Work out the finished part from the listing and answer in its coordinate system (mm). A direction names the side the tool comes from. Round coordinates to 2 decimals unless told otherwise and drop trailing zeros. Loops run counter-clockwise (first coordinate to the right, second up) from the corner with the lowest first, then second, coordinate; pieces in that order, holes last. Notation, with made-up numbers: (69, 23) - (75, 23) arc R16 cw to (75, 34) - close; hole circle Ø5 at (32.25, 22.25). An arc over 180 degrees is marked (long way). Return JSON: item names as keys, results as strings.
from build123d import *

# Parameters (mm, degrees)
F0_W     = 10
F0_H     = 20
F1_DEPTH = 1.5
F2_W     = 10
F2_H     = 1.5
F3_DEPTH = 18.5
F5_DEPTH = 1.501
F7_DEPTH = 1.501
F9_DEPTH = 1
F10_R    = 0.99999


# Not quite as in the source:
# - a fillet or chamfer is up to 0.001 mm smaller than in the source, because OpenCascade refuses the exact size
# - a pattern or mirror of a feature is missing from the dataset's text; its kind, count and spacing are read off the source's solid


with BuildPart() as f1:
    # F0 (on Top) → F1 (new body)
    with BuildSketch(Plane.XY):
        Rectangle(F0_W, F0_H)
    extrude(amount=F1_DEPTH)

    # F2 (on face) → F3 (join)
    with BuildSketch(Plane.XY.offset(1.5)):
        with Locations((0, 9.25)):
            Rectangle(F2_W, F2_H)
    extrude(amount=F3_DEPTH)

    # F4 (on face) → F5 (cut, through all)
    with BuildSketch(Plane.XY.offset(1.5)):
        with BuildLine():
            ThreePointArc((0, -5), (1.2727922061, -4.4727922061), (1.8, -3.2))
            Line((1.8, -3.2), (1.8, 3.2))
            ThreePointArc((1.8, 3.2), (1.2727922061, 4.4727922061), (0, 5))
            ThreePointArc((0, 5), (-1.2727922061, 4.4727922061), (-1.8, 3.2))
            Line((-1.8, 3.2), (-1.8, -3.2))
            ThreePointArc((-1.8, -3.2), (-1.2727922061, -4.4727922061), (0, -5))
        make_face()
    extrude(amount=-F5_DEPTH, mode=Mode.SUBTRACT)

    # F6 (on face) → F7 (cut, through all)
    with BuildSketch(Plane.XZ.offset(-8.5)):
        with BuildLine():
            ThreePointArc((0, 4.6788305809), (1.2727922061, 5.2060383747), (1.8, 6.4788305809))
            Line((1.8, 6.4788305809), (1.8, 12.8788305809))
            ThreePointArc((1.8, 12.8788305809), (1.2727922061, 14.151622787), (0, 14.6788305809))
            ThreePointArc((0, 14.6788305809), (-1.2727922061, 14.151622787), (-1.8, 12.8788305809))
            Line((-1.8, 12.8788305809), (-1.8, 6.4788305809))
            ThreePointArc((-1.8, 6.4788305809), (-1.2727922061, 5.2060383747), (0, 4.6788305809))
        make_face()
    extrude(amount=-F7_DEPTH, mode=Mode.SUBTRACT)

    # F8 (on face) → F9 (join)
    with BuildSketch(Plane(origin=(-5, 0, 0), x_dir=(0, -1, 0), z_dir=(-1, 0, 0))):
        Polygon((10, 1.5), (-8.5, 20), (-8.5, 1.5), align=None)
    f9 = extrude(amount=-F9_DEPTH)

    # F9_copies: F9 across plane
    add(f9.mirror(Plane(origin=(0, 0, 0), x_dir=(0, 0, 1), z_dir=(1, 0, 0))))

    # F10 (radius 1 in the source; OpenCascade refuses exactly that, so slightly less here)
    f10_edges = [f1.edges().sort_by_distance(p)[0] for p in [
        (-5, -0.75, 10.75),
        (5, -0.75, 10.75),
    ]]
    fillet(f10_edges, radius=F10_R)


solid = f1.part
1) Section A-A (x = -2.5) is taken. Give the vertices of the cut face in (y, z), and give its area (4 significant figures).
Verdict:
{"outline": "(-10, 0) - (10, 0) - (10, 20) - (8.5, 20) - (8.5, 1.5) - (-10, 1.5) - close", "area": "57.75 mm2"}
2) Section B-B (x = -0.5) is taken. Give the vertices of the cut face in (y, z).
Verdict:
{"outline": "(-10, 0) - (-4.93, 0) - (-4.93, 1.5) - (-10, 1.5) - close; (4.93, 0) - (10, 0) - (10, 4.75) - (8.5, 4.75) - (8.5, 1.5) - (4.93, 1.5) - close; (8.5, 14.61) - (10, 14.61) - (10, 20) - (8.5, 20) - close"}
3) Determine the mould class of faces 4 (the flat face through (-1.8, 0, 1)), 5 (the flat face through (-1.8, 9, 10)), 6 (the flat face through (1.8, 9, 10)), 7 (the flat face through (-2, -1, 1.5)) for opening direction Z: pulls with the +Z half, pulls with the -Z half, needs draft (parallel to the pull), parting line crosses it, or undercut.
Verdict:
{"face 4": "needs draft", "face 5": "undercut", "face 6": "undercut", "face 7": "pulls with the +Z half"}
4) Find the intervals of material crossed by L1, parallel to X at y = 7, z = 11.75; L2, parallel to Z at x = -1.75, y = -5.75; L3, parallel to Y at x = -2.5, z = 6.5, in increasing order.
Verdict:
{"L1": "x = -5 to -4, 4 to 5", "L2": "z = 0 to 1.5", "L3": "y = 8.5 to 10"}
5) A flat-ended cylindrical pin translates along its axis: pin 1 (3 mm diameter, centred on x = -0.5, z = 11, fed in from -Y). Find the tip coordinate at first contact, or state that the pin passes through.
Verdict:
{"pin 1": "stops at y = 8.5"}
6) A tool of negligible diameter and unlimited length cuts with its end or side. For faces 1 (the flat face through (1.8, 0, 1)), 2 (the flat face through (-2, 10, 10)), 3 (the flat face through (-2, 8.5, 11)), from which of +Z, -Z, +X, -X, +Y, -Y can it reach the whole face along a straight path? Write none if from no direction.
Verdict:
{"face 1": "+Z, -Z", "face 2": "+Z, -Z, +X, -X, +Y", "face 3": "+Z, -Y"}
